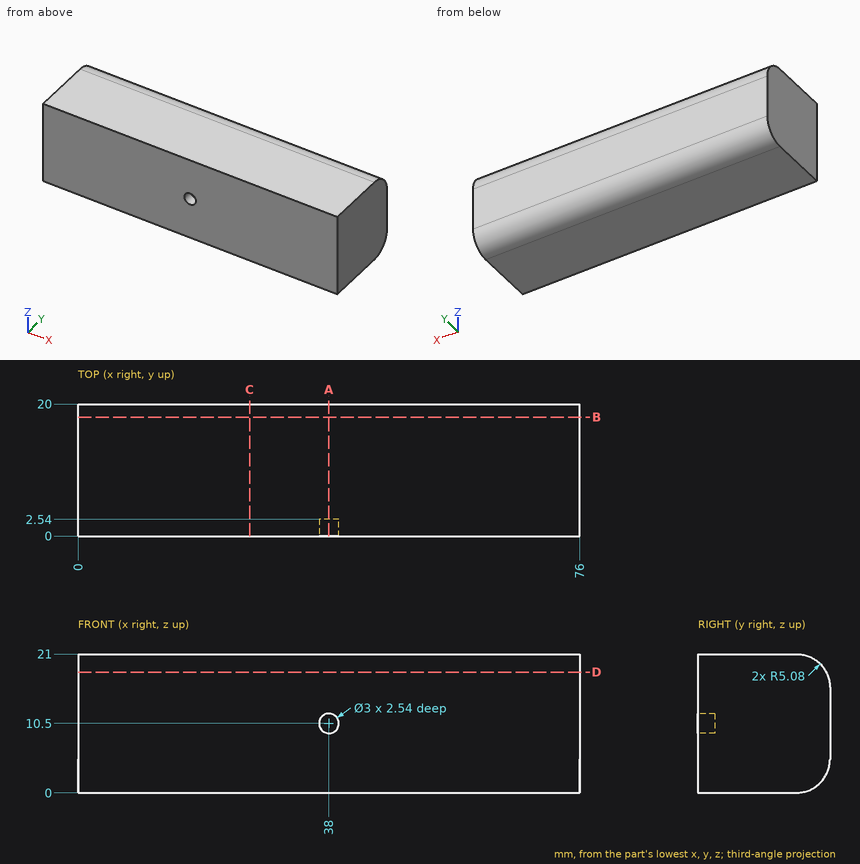
Answer from the drawing. Dimensions are ordinates in mm from the lowest x, y and z of the part. Coordinates: 2 decimals unless noted, no trailing zeros. Write each loop counter-clockwise with the first axis right and the second up, starting at its lowest first coordinate (ties: lowest second). Pieces come first, ordered by that corner, then holes. Notation, with made-up numbers: M 76.5,-28 L 101.5,-28 A24 ccw 101.5,2 Z; hole C 30,70 d9. An arc over 180 degrees is marked long. Use a Markdown table: item, result.
Q1. This flat-tipped pin is pushed along its axis until it touches: pin 1 Ø1.5 at (x, z) = (37.5, 10.5) entering from -Y. Where does it stop, or does it pass through?
Answer block:
| item | result |
|---|---|
| pin 1 | stops at y = 2.54 |
Q2. The part is cut by section B-B, the plane y = 18. Write down the section's boundary in (x, z), then the cut area to 3 significant figures.
Answer block:
| item | result |
|---|---|
| outline | M 0,1.04 L 76,1.04 L 76,19.96 L 0,19.96 Z |
| area | 1,440 mm2 |
Q3. Straight lines are drawn through the part: L1, parallel to Z at x = 38, y = 1.2; L2, parallel to Y at x = 13, z = 5; L3, parallel to Y at x = 64, z = 4. For each, find the intervals that lie inside material, in ascending order. Write a range as [from, to].
Answer block:
| item | result |
|---|---|
| L1 | z = [0, 9], [12, 21] |
| L2 | y = [0, 20] |
| L3 | y = [0, 19.88] |
Q4. The part is cut by section C-C, the plane x = 26. Write down the section's boundary in (y, z).
Answer block:
| item | result |
|---|---|
| outline | M 0,0 L 14.92,0 A5.08 ccw 20,5.08 L 20,15.92 A5.08 ccw 14.92,21 L 0,21 Z |
Q5. The part is cut by section A-A, the plane x = 38. Write down the section's boundary in (y, z).
Answer block:
| item | result |
|---|---|
| outline | M 0,0 L 14.92,0 A5.08 ccw 20,5.08 L 20,15.92 A5.08 ccw 14.92,21 L 0,21 L 0,12 L 2.54,12 L 2.54,9 L 0,9 Z |
Q6. The part is cut by section D-D, the plane z = 18.25. Write down the section's boundary in (x, y), then the cut area to 3 significant figures.
Answer block:
| item | result |
|---|---|
| outline | M 0,0 L 76,0 L 76,19.43 L 0,19.43 Z |
| area | 1,480 mm2 |
